from build123d import *

# Parameters (mm, degrees)
F3_SIZE = 2.54


# Not quite as in the source:
# - a fillet or chamfer that OpenCascade refuses, or shapes differently, is made with other operations: its cross-section is extruded or revolved along the edge and cut away or added


with BuildPart() as f1:
    # F0 (on Front) → F1 (revolve)
    with BuildSketch(Plane.XZ):
        Polygon((0, 2.484759083), (0, 0), (12.7, 0), (18.2904321501, 12.7), (16.0741669896, 12.7), (11.577504687, 2.484759083), align=None)
    revolve(axis=Axis((0, 0, 10.5566112325), (0, 0, 1)))

    # F2: fillet of radius 2.0499963011 on 1 edges, made by hand

    # F2_s1 → F2_t2 (revolve, cut)
    with BuildSketch(Plane.XZ):
        with BuildLine():
            ThreePointArc((17.1048272979, 10.0066158002), (17.1431716206, 11.5651790127), (16.0741669896, 12.7))
            Line((16.0741669896, 12.7), (18.2904321501, 12.7))
            Line((18.2904321501, 12.7), (17.1048272979, 10.0066158002))
        make_face()
    revolve(axis=Axis((0, 0, 12.7), (0, 0, 1)), mode=Mode.SUBTRACT)

    # F3
    f3_edges = [f1.edges().sort_by_distance(p)[0] for p in [
        (-12.7, 0, 0),
    ]]
    chamfer(f3_edges, length=F3_SIZE)


solid = f1.part
Could you check a few things on this model? Use its own coordinates, in mm. Give positions to 0.01 mm unless a question says otherwise; leave off trailing zeros. Order: outer loops, then holes, each group sorted by start corner. A loop starts at its lowest first (then second) coordinate and runs counter-clockwise, first axis right, second up.
1. For pin 1 (1 mm diameter, centred on x = -11, y = 4.5, fed in from +Z); pin 2 (4 mm diameter, centred on x = -2.5, z = 4.5, fed in from +Y); pin 3 (6 mm diameter, centred on x = 3.5, y = -8, fed in from -Z); pin 4 (3 mm diameter, centred on x = -2.5, y = -8, fed in from +Z), each with a flat end and sliding along its axis, tell me the tip position at first contact or that it passes through.
Answers below:
pin 1: stops at z = 4.32
pin 2: stops at y = 15.4
pin 3: stops at z = 0
pin 4: stops at z = 2.48
2. Suppose I cut it at C-C (z = 4). Write out the boundary of the cut face in (x, y).
Answers below:
outline: circle Ø28.92 at (0, 0); hole circle Ø24.49 at (0, 0)
3. Suppose I cut it at A-A (y = 0). Write out the boundary of the cut face in (x, z), plus the area to 3 significant figures.
Answers below:
outline: (-17.1, 10.01) - (-13.72, 2.32) - (-10.16, 0) - (10.16, 0) - (13.72, 2.32) - (17.1, 10.01) arc R2.05 ccw to (16.07, 12.7) - (11.58, 2.48) - (-11.58, 2.48) - (-16.07, 12.7) arc R2.05 ccw to start
area: 102 mm2
4. Thinking about a two-plate mould opening in X: for faces 1 (the conical face through (-3.021, -13.603, 2.805)), 2 (the flat face through (0, 0, 2.485)), 3 (the flat face through (0, 0, 0)), which applies, +X half, -X half, draft (parallel to the pull), parting line (faces both ways), or undercut?
Answers below:
face 1: parting line
face 2: undercut
face 3: draft
5. I need wall thicknesses on L1, parallel to Z at x = -0.5, y = 9; L2, parallel to Y at x = 2.5, z = 6.75; L3, parallel to Y at x = -9.5, z = 10.5. Which ranges of each line are inside material? Lowest first, please.
Answers below:
L1: z = 0 to 2.48
L2: y = -15.47 to -13.22, 13.22 to 15.47
L3: y = -14.4 to -11.74, 11.74 to 14.4
6. Suppose I cut it at D-D (z = 1.75). Write out the boundary of the cut face in (x, y).
Answers below:
outline: circle Ø25.68 at (0, 0)
